Design review of the part built by this model. Coordinates are the model's own, in mm. A direction names the side the tool comes from. Coordinates: 2 decimals unless noted, no trailing zeros. Write each loop counter-clockwise with the first axis right and the second up, starting at its lowest first coordinate (ties: lowest second). Pieces come first, ordered by that corner, then holes. Notation, with made-up numbers: (78.5, 65) - (99.5, 65) arc R19 cw to (99.5, 101) - close; hole circle Ø8 at (13, -35.75). An arc over 180 degrees is marked (long way). Answer as CSV lines item,"result". Start each with the question number.
Q1. We need section D-D (x = -6.5). Write out the cut boundary in (y, z).
Q2. Clearance check with flat-ended pins moving along their axes: pin 1 (4 mm diameter, centred on y = 16, z = 13, fed in from -X); pin 2 (7.5 mm diameter, centred on y = 14.5, z = -7, fed in from +X); pin 3 (1.5 mm diameter, centred on x = 6, y = 3.5, fed in from -Z). State where each tip first meets the part, or that it passes through.
Q3. Machinability: for faces 1 (the face through (2, 2, -12.5)), 2 (the face through (1, 2, 12.5)), 3 (the face through (5, 5, 0)), which of the approach directions +Z, -Z, +X, -X, +Y, -Y give a long, thin tool a straight path to every point of the face, cutting with its end or side? Answer none if there is none.
Q4. We need section C-C (z = -9.5). Write out the cut boundary in (x, y), plus the area to 3 significant figures.
Q5. Mouldability with a two-part tool opening along Z and no side actions: class faces 4 (the face through (-1.5, 3.52, 2.54)), 5 (the face through (-8.5, 15, 0)), 6 (the face through (-14, 12, 10)) as pulls with the +Z half, pulls with the -Z half, needs draft (parallel to the pull), parting line crosses it, or undercut.
Q6. For line 1 along Z through (x, y) = (0, 1.45); line 2 along X through (y, z) = (8, 5.25); line 3 along Y through (x, z) = (1.5, 8.5), list the stretches that pass through material, from the lowest coordinate up. Write a range as [from, to].
Q7. We need section A-A (z = 0). Write out the cut boundary in (x, y).
Q8. We need section B-B (y = 20.5). Write out the cut boundary in (x, z), plus the area to 3 significant figures.
from build123d import *

# Parameters (mm, degrees)
BOSS_EXTRUDE1_DEPTH     = 5
BOSS_EXTRUDE2_DEPTH     = 20
CUT_EXTRUDE1_DEPTH      = 34.018933962
CUT_EXTRUDE1_DEPTH_BACK = 34.018933962
SKETCH4_R               = 2.5
FILLET1_R               = 1
FILLET2_R               = 1
FILLET3_R               = 2
CUT_EXTRUDE2_DEPTH      = 3


with BuildPart() as part:
    # Sketch2 → Boss-Extrude1 (new body)
    with BuildSketch(Plane(origin=(0, 0, 0), x_dir=(1, 0, 0), z_dir=(0, 1, 0))):
        Polygon((-8.5, -12.5), (12.5, -12.5), (12.5, 12.5), (-8.5, 12.5), (-8.5, 15), (-12.5, 15), (-12.5, 10), (-15.5, 10), (-15.5, -10), (-12.5, -10), (-12.5, -15), (-8.5, -15), align=None)
    extrude(amount=BOSS_EXTRUDE1_DEPTH)

    # Sketch3 → Boss-Extrude2 (add)
    with BuildSketch(Plane(origin=(0, 5, 0), x_dir=(1, 0, 0), z_dir=(0, 1, 0))):
        Polygon((-15.5, 10), (-15.5, -10), (-12.5, -10), (-12.5, -15), (-8.5, -15), (-8.5, 15), (-12.5, 15), (-12.5, 10), align=None)
    extrude(amount=BOSS_EXTRUDE2_DEPTH)

    # Sketch4 → Cut-Extrude1 (cut, two sides: drawn at the far end of the back side and taken through both)
    with BuildSketch(Plane.XZ.offset(-CUT_EXTRUDE1_DEPTH_BACK)):
        with Locations(Location((0, 0, 0), (0, 0, 270))):
            Circle(SKETCH4_R)
    extrude(amount=CUT_EXTRUDE1_DEPTH + CUT_EXTRUDE1_DEPTH_BACK, mode=Mode.SUBTRACT)

    # Fillet1
    fillet1_edges = [part.edges().sort_by_distance(p)[0] for p in [
        (0, 0, 2.5),
    ]]
    fillet(fillet1_edges, radius=FILLET1_R)

    # Fillet2
    fillet2_edges = [part.edges().sort_by_distance(p)[0] for p in [
        (-8.5, 2.5, -12.5),
        (-8.5, 2.5, 12.5),
        (-8.5, 5, 0),
    ]]
    fillet(fillet2_edges, radius=FILLET2_R)

    # Fillet3
    fillet3_edges = [part.edges().sort_by_distance(p)[0] for p in [
        (12.5, 0, 0),
        (12.5, 2.5, -12.5),
        (12.5, 2.5, 12.5),
    ]]
    fillet(fillet3_edges, radius=FILLET3_R)

    # Sketch5 → Cut-Extrude2 (cut)
    with BuildSketch(Plane(origin=(0, 5, 0), x_dir=(1, 0, 0), z_dir=(0, 1, 0))):
        Polygon((2.95, 1.703183294), (0, 3.406366588), (-2.95, 1.703183294), (-2.95, -1.703183294), (0, -3.406366588), (2.95, -1.703183294), align=None)
    extrude(amount=-CUT_EXTRUDE2_DEPTH, mode=Mode.SUBTRACT)


solid = part.part
Results list:
1,outline,"(0, -12.5) - (5, -12.5) - (5, 12.5) - (0, 12.5) - close"
2,pin 1,"stops at x = -12.5"
2,pin 2,"stops at x = -8.5"
2,pin 3,"stops at z = -12.5"
3,face 1,"-Z, +X, +Y, -Y"
3,face 2,"+Z, +X, +Y, -Y"
3,face 3,"+Z, -Z, +X, +Y"
4,outline,"(-15.5, 0) - (10.5, 0) arc R2 ccw to (12.5, 2) - (12.5, 5) - (-7.5, 5) arc R1 cw to (-8.5, 6) - (-8.5, 25) - (-15.5, 25) - close"
4,area,"279 mm2"
5,face 4,"undercut"
5,face 5,"needs draft"
5,face 6,"pulls with the +Z half"
6,line 1,"z = [-12.5, -2.5], [2.5, 12.5]"
6,line 2,"x = [-15.5, -8.5]"
6,line 3,"y = [0, 5]"
7,outline,"(-15.5, 0) - (-3.5, 0) arc R1 ccw to (-2.5, 1) - (-2.5, 2) - (-2.95, 2) - (-2.95, 5) - (-7.5, 5) arc R1 cw to (-8.5, 6) - (-8.5, 25) - (-15.5, 25) - close; (2.5, 1) arc R1 ccw to (3.5, 0) - (10.5, 0) arc R2 ccw to (12.5, 2) - (12.5, 5) - (2.95, 5) - (2.95, 2) - (2.5, 2) - close"
8,outline,"(-15.5, -10) - (-12.5, -10) - (-12.5, -15) - (-8.5, -15) - (-8.5, 15) - (-12.5, 15) - (-12.5, 10) - (-15.5, 10) - close"
8,area,"180 mm2"
